Autodesk Inventor part; units mm, degrees
ref_plane "YZ Plane" through (0, 0, 0) normal (1, 0, 0) x (0, 1, 0)
ref_plane "XZ Plane" through (0, 0, 0) normal (0, 1, 0) x (-1, 0, 0)
ref_plane "XY Plane" through (0, 0, 0) normal (0, 0, 1) x (1, 0, 0)
sketch "Sketch2" plane through (0, 0, 0) normal (0, 0, 1) x (1, 0, 0)
  line L0 (-54, -101) -> (54, -101)
  line L1 (54, -101) -> (54, 101)
  line L2 (54, 101) -> (-54, 101)
  line L3 (-54, 101) -> (-54, -101)
  line L4 (-54, -101) -> (54, 101) construction
  line L5 (54, -101) -> (-54, 101) construction
  line L6 (-104, -151) -> (104, -151)
  line L7 (104, -151) -> (104, 151)
  line L8 (104, 151) -> (-104, 151)
  line L9 (-104, 151) -> (-104, -151)
  point P0 (0, 0)
  dimension "d29" = 108
  dimension "d30" = 202
  dimension "d31" = 50
  dimension "d47" = 208
  dimension "d48" = 302
extrude "Plate2" add sketch "Sketch2" along normal blind 10
sketch "Sketch5" plane through (0, 0, 10) normal (0, 0, 1) x (1, 0, 0)
  line L0 (54, 101) -> (54, -101) construction
  line L1 (54, -101) -> (-54, -101) construction
  line L2 (-54, -101) -> (-54, 101) construction
  line L3 (-54, 101) -> (54, 101) construction
  line L4 (104, -151) -> (-104, -151) construction
  line L5 (104, 151) -> (104, -151) construction
  line L6 (-104, 151) -> (104, 151) construction
  line L7 (-104, -151) -> (-104, 151) construction
  line L8 (-85, 132) -> (85, 132) construction
  line L9 (85, 132) -> (85, -132) construction
  line L10 (85, -132) -> (-85, -132) construction
  line L11 (-85, -132) -> (-85, 132) construction
  circle A0 centre (-85, -132) radius 8.5
  circle A1 centre (-85, 132) radius 8.5
  circle A2 centre (-85, 0) radius 8.5
  circle A3 centre (-85, -66) radius 8.5
  circle A4 centre (-85, 66) radius 8.5
  line L12 (-54, 0) -> (54, 0) construction
  circle A5 centre (-31, -132) radius 8.5
  circle A6 centre (-31, -66) radius 8.5
  circle A7 centre (-31, 0) radius 8.5
  circle A8 centre (-31, 66) radius 8.5
  circle A9 centre (-31, 132) radius 8.5
  circle A10 centre (23, -132) radius 8.5
  circle A11 centre (23, -66) radius 8.5
  circle A12 centre (23, 0) radius 8.5
  circle A13 centre (23, 66) radius 8.5
  circle A14 centre (23, 132) radius 8.5
  circle A15 centre (77, -132) radius 8.5
  circle A16 centre (77, -66) radius 8.5
  circle A17 centre (77, 0) radius 8.5
  circle A18 centre (77, 66) radius 8.5
  circle A19 centre (77, 132) radius 8.5
  point P0 (0, 0)
  point P1 (0, -132)
  dimension "d33" = 17
  dimension "d34" = 19
  dimension "d35" = 66
  dimension "d36" = 66
  dimension "d39" = 54
extrude "Cut3" cut sketch "Sketch5" against normal blind 10
fillet "Corner Round1" radius 6 8 edges at (-104, -151, 5) (-104, 151, 5) (104, 151, 5) (104, -151, 5) (54, -101, 5) (-54, -101, 5) (-54, 101, 5) (54, 101, 5)
equation "\"d35\" = d36"
equation "\"d44\" = Thickness"
equation "\"d14\" = Thickness"
equation "\"BendReliefDepth\" = 0.5 * Thickness"
equation "\"TransitionRadius\" = BendRadius"
equation "\"JacobiRadiusSize\" = BendRadius"
properties part number "PRS 1200-06 charging flange round" material "Steel"
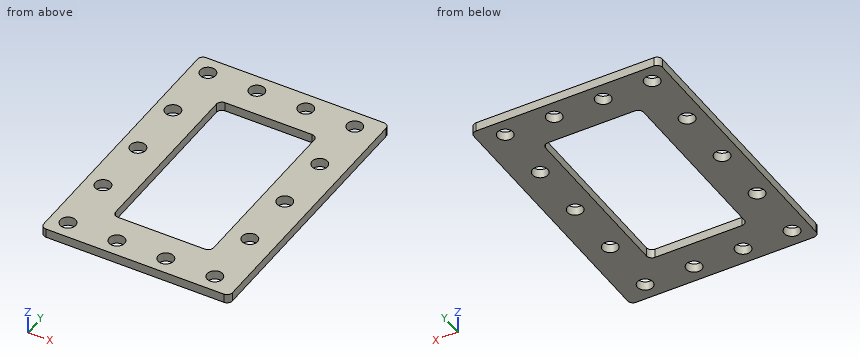
The listing builds one solid part. Answer for the finished solid, in the listing's coordinates (mm). Coordinates: 2 decimals unless noted, no trailing zeros. Loops run counter-clockwise (first coordinate to the right, second up) from the corner with the lowest first, then second, coordinate; pieces in that order, holes last. Notation, with made-up numbers: (-35, 87.25) -> (12, 87.25) arc R32 cw to (12, 116.25) -> close; hole circle Ø7 at (-15.5, 17). An arc over 180 degrees is marked (long way). Use one line per item in the form item = value. Start each with the question number.
Item 1: The part is cut by section B-B on y = 83. Determine the outline of the cut face in (x, z).
Item 2: The part is cut by section A-A on x = 41. Determine the outline of the cut face in (y, z).
Item 3: The part is cut by section C-C on z = 8.25. Count the separate pieces of the cut face and the enclosed holes in it, then the cut area to 3 significant figures.
Item 4: The part is cut by section D-D on y = -132. Determine the outline of the cut face in (x, z).
Item 5: Consider L1, parallel to Y at x = 77, z = 3.25; L2, parallel to Y at x = -31, z = 4.5; L3, parallel to X at y = 81.5, z = 4. Determine where each line is inside the solid, lowest interval first. Write a range as [from, to].
Answer key:
q1.outline = (-104, 0) -> (-54, 0) -> (-54, 10) -> (-104, 10) -> close; (54, 0) -> (104, 0) -> (104, 10) -> (54, 10) -> close
q2.outline = (-151, 0) -> (-101, 0) -> (-101, 10) -> (-151, 10) -> close; (101, 0) -> (151, 0) -> (151, 10) -> (101, 10) -> close
q3.separate_pieces = 1
q3.enclosed_holes = 15
q3.area = 37,800 mm2
q4.outline = (-104, 0) -> (-93.5, 0) -> (-93.5, 10) -> (-104, 10) -> close; (-76.5, 0) -> (-39.5, 0) -> (-39.5, 10) -> (-76.5, 10) -> close; (-22.5, 0) -> (14.5, 0) -> (14.5, 10) -> (-22.5, 10) -> close; (31.5, 0) -> (68.5, 0) -> (68.5, 10) -> (31.5, 10) -> close; (85.5, 0) -> (104, 0) -> (104, 10) -> (85.5, 10) -> close
q5.L1 = [-151, -140.5], [-123.5, -74.5], [-57.5, -8.5], [8.5, 57.5], [74.5, 123.5], [140.5, 151]
q5.L2 = [-151, -140.5], [-123.5, -101], [101, 123.5], [140.5, 151]
q5.L3 = [-104, -54], [54, 104]
